Drawing for the job (mm, zero at the part's lowest x, y, z). A direction names the side the tool comes from. Give positions to 0.01 mm unless a question says otherwise; leave off trailing zeros. Order: outer loops, then holes, each group sorted by start corner. A loop starts at its lowest first (then second) coordinate and runs counter-clockwise, first axis right, second up. Notation, with made-up numbers: (62, 5) - (91, 5) arc R14 ccw to (91, 10) - close; hole circle Ø4 at (-27.5, 43.25). An arc over 180 degrees is marked (long way). Use CSV: the item, a comma, the result in double quotes. Start each with the question number.
(1) Band-saw the part on A-A, the plane z = 5. Give the cut face in (x, y), then the cut area to 3 significant figures.
(2) Tool access for the marked faces 4, 5, 6 and 7: list every direction of +Z, -Z, +X, -X, +Y, -Y with a clear straight run to the whole face (end or side of a thin tool).
(3) Band-saw the part on B-B, the plane y = 15. Give the cut face in (x, z).
(4) Band-saw the part on C-C, the plane x = 15. Give the cut face in (y, z), then the cut area to 3 significant figures.
(5) Band-saw the part on D-D, the plane y = 26.5. Give the cut face in (x, z), then the cut area to 3 significant figures.
(6) Pull direction Y, two halves, no side cores. Call the marked faces 1, 2 and 3: +Y half, -Y half, draft (parallel to the pull), parting line (faces both ways), or undercut.
(7) Probe L1, parallel to Y at x = 15, z = 23.55; L2, parallel to Z at x = 22, y = 19; L3, parallel to Y at x = 9.5, z = 8.25. List the from-to ranges inside material, lowest first.
(8) Drop flat-ended pins along their axis: pin 1 Ø1.3 at (x, z) = (17.5, 28.5) entering from +Y; pin 2 Ø12 at (y, z) = (17.5, 22.5) entering from -X; pin 3 Ø1 at (y, z) = (29, 11.5) entering from -X; pin 4 Ø9 at (x, y) = (16, 14.5) entering from +Z. Give the stop position or say it passes through.
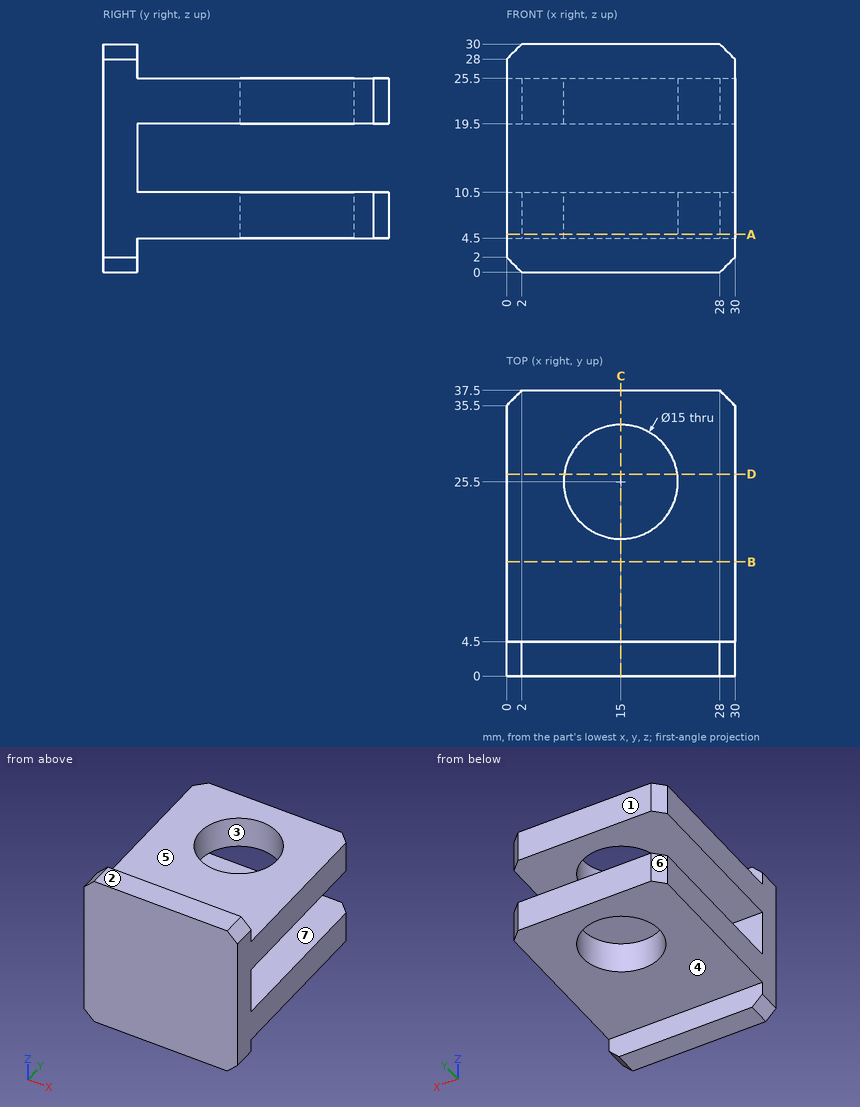
Answer block:
1,outline,"(0, 0) - (30, 0) - (30, 35.5) - (28, 37.5) - (2, 37.5) - (0, 35.5) - close; hole circle Ø15 at (15, 25.5)"
1,area,"944 mm2"
2,face 4,"-Z, +X, -X, +Y"
2,face 5,"+Z, +X, -X, +Y"
2,face 6,"+Z, -Z, -X, +Y"
2,face 7,"+X, -X, +Y"
3,outline,"(0, 4.5) - (30, 4.5) - (30, 10.5) - (0, 10.5) - close; (0, 19.5) - (30, 19.5) - (30, 25.5) - (0, 25.5) - close"
4,outline,"(0, 0) - (4.5, 0) - (4.5, 4.5) - (18, 4.5) - (18, 10.5) - (4.5, 10.5) - (4.5, 19.5) - (18, 19.5) - (18, 25.5) - (4.5, 25.5) - (4.5, 30) - (0, 30) - close; (33, 4.5) - (37.5, 4.5) - (37.5, 10.5) - (33, 10.5) - close; (33, 19.5) - (37.5, 19.5) - (37.5, 25.5) - (33, 25.5) - close"
4,area,"351 mm2"
5,outline,"(0, 4.5) - (7.57, 4.5) - (7.57, 10.5) - (0, 10.5) - close; (0, 19.5) - (7.57, 19.5) - (7.57, 25.5) - (0, 25.5) - close; (22.43, 4.5) - (30, 4.5) - (30, 10.5) - (22.43, 10.5) - close; (22.43, 19.5) - (30, 19.5) - (30, 25.5) - (22.43, 25.5) - close"
5,area,"182 mm2"
6,face 1,"+Y half"
6,face 2,"draft"
6,face 3,"undercut"
7,L1,"y = 0 to 18, 33 to 37.5"
7,L2,"z = 4.5 to 10.5, 19.5 to 25.5"
7,L3,"y = 0 to 20.4, 30.6 to 37.5"
8,pin 1,"stops at y = 4.5"
8,pin 2,"stops at x = 0"
8,pin 3,"passes through"
8,pin 4,"stops at z = 25.5"
